```python
from build123d import *

# Parameters (mm, degrees)
SKETCH_1_R                     = 45
EXTRUDE_1_DEPTH                = 40
REVOLVE_1_ANGLE                = 180
CUT_EXTRUDE_2_DEPTH            = 107.183802908
CUT_EXTRUDE_2_DEPTH_BACK       = 107.183802908
SKETCH_8_R                     = 29.5
EXTRUDE_2_DEPTH                = 6
CUT_EXTRUDE_5_DEPTH            = 124.830529354
CUT_EXTRUDE_5_DEPTH_BACK       = 124.830529354
SKETCH_9_W                     = 18
SKETCH_9_H                     = 55
SKETCH_9_W_2                   = 20
SKETCH_9_H_2                   = 39.84
SKETCH_9_4_W                   = 7.65
SKETCH_9_4_H                   = 7.58
SKETCH_9_4_R                   = 1.5
EXTRUDE_3_DEPTH                = 4
SKETCH_9_5_W                   = 2.7
SKETCH_9_5_H                   = 7.58
EXTRUDE_4_DEPTH                = 2
HOLE_WIZARD_M3_1_D             = 2.5
CUT_EXTRUDE_6_DEPTH            = 107.183802908
CUT_EXTRUDE_6_DEPTH_BACK       = 107.183802908
SKETCH_10_OUTSIDE_W            = 123.292
SKETCH_10_OUTSIDE_H            = 123.292
SKETCH_10_OUTSIDE_R            = 45
SKETCH_14_R                    = 2.5
EXTRUDE_5_DEPTH                = 2.5
EXTRUDE_6_DEPTH                = 15
HOLE_WIZARD_M3_1_2_D           = 8
HOLE_WIZARD_M3_1_2_CBORE_D     = 9.5
HOLE_WIZARD_M3_1_2_CBORE_DEPTH = 0.9
SKETCH_23_R                    = 5
CUT_EXTRUDE_8_DEPTH            = 124.830529354
EXTRUDE_START                  = -36
EXTRUDE_7_OUTLINE_R            = 5
EXTRUDE_7_DEPTH                = 4
HOLE_WIZARD_M5_1_D             = 8
HOLE_WIZARD_M5_1_DEPTH         = 10
HOLE_WIZARD_M5_1_CBORE_D       = 9.5
HOLE_WIZARD_M5_1_CBORE_DEPTH   = 0.9
HOLE_WIZARD_M5_1_TIP           = 2.403442476
CHAMFER_1_SIZE                 = 1


# Read off the part's stored shape, not the designer's step: 凸台-拉伸7
with BuildPart() as part:
    # 草图1 → 凸台-拉伸1 (new body)
    with BuildSketch(Plane(origin=(0, 0, 0), x_dir=(1, 0, 0), z_dir=(0, 1, 0))):
        with Locations(Location((0, 0, 0), (0, 0, 270))):
            Circle(SKETCH_1_R)
    extrude(amount=EXTRUDE_1_DEPTH)

    # 草图3 → 旋转1 (revolve)
    with BuildSketch(Plane(origin=(0, 40, 0), x_dir=(1, 0, 0), z_dir=(0, 1, 0))):
        with BuildLine():
            ThreePointArc((45, 0), (31.819805153, 31.819805153), (0, 45))
            Line((0, 45), (0, 0))
            Line((0, 0), (45, 0))
        make_face()
        with BuildLine():
            Line((45, 0), (0, 0))
            Line((0, 0), (0, -45))
            ThreePointArc((0, -45), (31.819805153, -31.819805153), (45, 0))
        make_face()
        with BuildLine():
            Line((45, 45), (0, 45))
            ThreePointArc((0, 45), (31.819805153, 31.819805153), (45, 0))
            Line((45, 0), (45, 45))
        make_face()
        with BuildLine():
            Line((45, -45), (45, 0))
            ThreePointArc((45, 0), (31.819805153, -31.819805153), (0, -45))
            Line((0, -45), (45, -45))
        make_face()
    revolve(axis=Axis((0, 40, -45), (0, 0, 1)), revolution_arc=REVOLVE_1_ANGLE)

    # 草图4 → 切除-拉伸2 (cut, two sides: drawn at the far end of the back side and taken through both)
    with BuildSketch(Plane(origin=(0, 0, 0), x_dir=(0, 0, -1), z_dir=(1, 0, 0)).offset(-CUT_EXTRUDE_2_DEPTH_BACK)):
        Polygon((33, 162), (-33, 162), (-33, 14.4), (-33, 8), (-26.603931708, 8), (26.603931708, 8), (33, 8), (33, 14.4), align=None)
    extrude(amount=CUT_EXTRUDE_2_DEPTH + CUT_EXTRUDE_2_DEPTH_BACK, mode=Mode.SUBTRACT)

    # 草图8 → 凸台-拉伸2 (add)
    with BuildSketch(Plane.XZ):
        with Locations(Location((0, 0, 0), (0, 0, 270))):
            Circle(SKETCH_8_R)
    extrude(amount=EXTRUDE_2_DEPTH)

    # 草图9 → 切除-拉伸5 (cut, two sides: drawn at the far end of the back side and taken through both)
    with BuildSketch(Plane.XY.offset(-33).offset(-CUT_EXTRUDE_5_DEPTH_BACK)):
        with Locations((0, 45)):
            Rectangle(SKETCH_9_W, SKETCH_9_H)
        with Locations((0, 45)):
            Rectangle(SKETCH_9_W_2, SKETCH_9_H_2)
    extrude(amount=CUT_EXTRUDE_5_DEPTH + CUT_EXTRUDE_5_DEPTH_BACK, mode=Mode.SUBTRACT)

    # 草图9<4> → 凸台-拉伸3 (add)
    # profile 1 of 4: a face of its own
    with BuildSketch(Plane.XY.offset(-33)):
        with Locations((5.175, 21.29)):
            Rectangle(SKETCH_9_4_W, SKETCH_9_4_H)
        with Locations((4.975, 20.47)):
            Circle(SKETCH_9_4_R, mode=Mode.SUBTRACT)
    # profile 2 of 4: a face of its own
    with BuildSketch(Plane.XY.offset(-33)):
        with Locations((-5.175, 21.29)):
            Rectangle(SKETCH_9_4_W, SKETCH_9_4_H)
        with Locations((-4.975, 20.47)):
            Circle(SKETCH_9_4_R, mode=Mode.SUBTRACT)
    # profile 3 of 4: a face of its own
    with BuildSketch(Plane.XY.offset(-33)):
        with Locations((5.175, 68.71)):
            Rectangle(SKETCH_9_4_W, SKETCH_9_4_H)
        with Locations((4.975, 69.53)):
            Circle(SKETCH_9_4_R, mode=Mode.SUBTRACT)
    # profile 4 of 4: a face of its own
    with BuildSketch(Plane.XY.offset(-33)):
        with Locations((-5.175, 68.71)):
            Rectangle(SKETCH_9_4_W, SKETCH_9_4_H)
        with Locations((-4.975, 69.53)):
            Circle(SKETCH_9_4_R, mode=Mode.SUBTRACT)
    extrude_3 = extrude(amount=-EXTRUDE_3_DEPTH)

    # 草图9<5> → 凸台-拉伸4 (add)
    with BuildSketch(Plane.XY.offset(-33)):
        with Locations((0, 21.29)):
            Rectangle(SKETCH_9_5_W, SKETCH_9_5_H)
        with Locations((0, 68.71)):
            Rectangle(SKETCH_9_5_W, SKETCH_9_5_H)
    extrude_4 = extrude(amount=-EXTRUDE_4_DEPTH)

    # 镜向1: 凸台-拉伸3, 凸台-拉伸4 across plane
    add(extrude_3.mirror(Plane.XY))
    add(extrude_4.mirror(Plane.XY))

    # Hole Wizard M3 _1 (through all)
    with Locations(Plane.XZ.offset(6)):
        with Locations((6.180339887, 19.021130326), (20, 0), (6.180339887, -19.021130326), (-16.180339887, -11.755705046), (-16.180339887, 11.755705046)):
            Hole(HOLE_WIZARD_M3_1_D / 2)

    # 草图10 outside → 切除-拉伸6 (cut, two sides: drawn at the far end of the back side and taken through both)
    with BuildSketch(Plane(origin=(0, 0, 0), x_dir=(1, 0, 0), z_dir=(0, 1, 0)).offset(-CUT_EXTRUDE_6_DEPTH_BACK)):
        Rectangle(SKETCH_10_OUTSIDE_W, SKETCH_10_OUTSIDE_H)
        with Locations(Location((0, 0, 0), (0, 0, 132.833428066))):
            Circle(SKETCH_10_OUTSIDE_R, mode=Mode.SUBTRACT)
    extrude(amount=CUT_EXTRUDE_6_DEPTH + CUT_EXTRUDE_6_DEPTH_BACK, mode=Mode.SUBTRACT)

    # 草图14 → 凸台-拉伸5 (add, symmetric)
    # profile 1 of 2: a face of its own
    with BuildSketch(Plane.XY):
        with BuildLine():
            Line((7.5, 35), (7.5, 8))
            Line((7.5, 8), (-7.5, 8))
            Line((-7.5, 8), (-7.5, 35))
            ThreePointArc((-7.5, 35), (0, 42.5), (7.5, 35))
        make_face()
        with Locations((0, 35)):
            Circle(SKETCH_14_R, mode=Mode.SUBTRACT)
    # profile 2 of 2: a face of its own
    with BuildSketch(Plane.XY):
        with Locations((0, 35)):
            Circle(SKETCH_14_R)
    extrude(amount=EXTRUDE_5_DEPTH, both=True)

    # 草图16 → 凸台-拉伸6 (add)
    with BuildSketch(Plane(origin=(7.5, 0, 0), x_dir=(0, 0, -1), z_dir=(1, 0, 0))):
        Polygon((2.5, 17.233050612), (5.5, 8), (2.5, 8), align=None)
    extrude_6 = extrude(amount=-EXTRUDE_6_DEPTH)

    # 镜向2: 凸台-拉伸6 across plane
    add(extrude_6.mirror(Plane.XY))

    # Hole Wizard M3 _1 2 (through all)
    with Locations(Plane.XY.offset(2.5)):
        with Locations((0, 35)):
            CounterBoreHole(HOLE_WIZARD_M3_1_2_D / 2, HOLE_WIZARD_M3_1_2_CBORE_D / 2, HOLE_WIZARD_M3_1_2_CBORE_DEPTH)

    # 草图23 → 切除-拉伸8 (cut, through all)
    with BuildSketch(Plane.XY.offset(-33)):
        with Locations((-20, 69.641016151)):
            Circle(SKETCH_23_R)
    extrude(amount=-CUT_EXTRUDE_8_DEPTH, mode=Mode.SUBTRACT)

    # 凸台-拉伸7 outline → 凸台-拉伸7 (add)
    with BuildSketch(Plane.XY.offset(EXTRUDE_START)):
        with Locations((-20, 69.641016151)):
            Circle(EXTRUDE_7_OUTLINE_R)
    extrude(amount=EXTRUDE_7_DEPTH)

    # M5 六角头螺栓的柱形沉头孔1
    with Locations(Plane(origin=(0, 0, -36), x_dir=(1, 0, 0), z_dir=(0, 0, -1))):
        with Locations((-20, -69.641016151)):
            CounterBoreHole(HOLE_WIZARD_M5_1_D / 2, HOLE_WIZARD_M5_1_CBORE_D / 2, HOLE_WIZARD_M5_1_CBORE_DEPTH, depth=HOLE_WIZARD_M5_1_DEPTH)
            with Locations((0, 0, -(HOLE_WIZARD_M5_1_DEPTH + HOLE_WIZARD_M5_1_TIP / 2))):  # 118° drill point
                Cone(0, HOLE_WIZARD_M5_1_D / 2, HOLE_WIZARD_M5_1_TIP, mode=Mode.SUBTRACT)

    # 倒角1
    chamfer_1_edges = [part.edges().sort_by_distance(p)[0] for p in [
        (-25, 69.641016151, -33),
    ]]
    chamfer(chamfer_1_edges, length=CHAMFER_1_SIZE - 0.0001)  # a hair under: the kernel refuses the full size


solid = part.part
```
Input: part model. Units: mm. Frame: model coordinates. A direction names the side the tool comes from. Give positions to 0.01 mm unless a question says otherwise; leave off trailing zeros. Write each loop counter-clockwise with the first axis right and the second up, starting at its lowest first coordinate (ties: lowest second). Pieces come first, ordered by that corner, then holes. Notation, with made-up numbers: (33.5, 61.5) - (82.5, 61.5) arc R25 ccw to (82.5, 98.5) - close; hole circle Ø7 at (16.25, 24.25). An arc over 180 degrees is marked (long way). Write item = value, one per line. Start each with the question number.
1) Cut plane D-D (x = 0). Give the number of separate pieces and of enclosed holes in the cut face, and give its area (3 significant figures).
2) Cut plane B-B (y = 14). Return loops of the section in (x, z).
3) Reachability of faces 1 (the face through (-7.5, 19, 0)), 2 (the face through (-6, 68, 37)), 3 (the face through (-24, 71, -35.1)), 4 (the face through (10, 45, 38)), 5 (the face through (0, 27, -2.5)) from +Z, -Z, +X, -X, +Y, -Y: full face, straight path, thin tool, end or side. Return the list, or none.
4) Material intervals for L1, parallel to Y at x = -12, z = 25; L2, parallel to Y at x = -12, z = -27; L3, parallel to X at y = -1.5, z = -19, sorted ascending. Write a range as [from, to].
5) Cut plane C-C (y = 78). Return loops of the section in (x, z).
6) Draft query along Z for faces 6 (the face through (8.86, -2.96, -28.14)), 7 (the face through (-9, 69, -41)), 8 (the face through (6.45, 1.1, -20.24)), 9 (the face through (0, 21, -35)). Return one class per face: pulls with the +Z half, pulls with the -Z half, needs draft (parallel to the pull), parting line crosses it, or undercut.
7) Pin query (flat end, axial travel): pin 1 (6.5 mm diameter, centred on x = -20, y = 69.64, fed in from -Z); pin 2 (8 mm diameter, centred on x = -4, z = -40.5, fed in from -Y); pin 3 (5 mm diameter, centred on x = -18.5, y = 69.5, fed in from +Z); pin 4 (6 mm diameter, centred on y = 26, z = -7, fed in from -X). Return the tip coordinate at first contact, or that it passes through.
Answers follow:
q1.separate_pieces = 4
q1.enclosed_holes = 0
q1.area = 1,820 mm^2
q2.outline = (-30.59, -33) arc R45 ccw to (30.59, -33) - close; (-30.59, 33) - (30.59, 33) arc R45 ccw to start; (-7.5, -3.55) - (7.5, -3.55) - (7.5, 3.55) - (-7.5, 3.55) - close
q3.face_1 = -X, +Y
q3.face_2 = +Z
q3.face_3 = -Z
q3.face_4 = +Z, -Z
q3.face_5 = +X, -X, +Y
q4.L1 = [-6, 8]
q4.L2 = [0, 8]
q4.L3 = [-22.57, 4.93], [7.43, 22.57]
q5.outline = (-24.1, -38) arc R45 ccw to (24.1, -38) - (24.1, -33) - (-24.1, -33) - close; (-24.1, 33) - (24.1, 33) - (24.1, 38) arc R45 ccw to (-24.1, 38) - close
q6.face_6 = parting line crosses it
q6.face_7 = needs draft
q6.face_8 = undercut
q6.face_9 = pulls with the -Z half
q7.pin_1 = 33
q7.pin_2 = 0
q7.pin_3 = 42.06
q7.pin_4 = through
